Model file for the job. Use its own axes, mm. Round coordinates to 2 decimals unless told otherwise and drop trailing zeros. Loops run counter-clockwise (first coordinate to the right, second up) from the corner with the lowest first, then second, coordinate; pieces in that order, holes last. Notation, with made-up numbers: (44, 49) -> (80, 49) arc R13 ccw to (80, 69) -> close; hole circle Ø1 at (27, 66.25). An arc over 180 degrees is marked (long way). Use a Markdown table: item, result.
Autodesk Inventor part; units mm, degrees
ref_plane "YZ Plane" through (0, 0, 0) normal (1, 0, 0) x (0, 1, 0)
ref_plane "XZ Plane" through (0, 0, 0) normal (0, 1, 0) x (-1, 0, 0)
ref_plane "XY Plane" through (0, 0, 0) normal (0, 0, 1) x (1, 0, 0)
sketch "Sketch1" plane through (0, 0, 0) normal (0, 0, 1) x (1, 0, 0)
  line L0 (3.6662, -6.35) -> (-3.6662, -6.35)
  line L1 (-3.6662, -6.35) -> (-7.3323, 0)
  line L2 (-7.3323, 0) -> (-3.6662, 6.35)
  line L3 (-3.6662, 6.35) -> (3.6662, 6.35)
  line L4 (3.6662, 6.35) -> (7.3323, 0)
  line L5 (7.3323, 0) -> (3.6662, -6.35)
  point P0 (0, 0)
  point P1 (0, 0)
  dimension "d0" = 12.7
extrude "Extrusion1" add sketch "Sketch1" along normal blind 161.925
sketch "Sketch2" plane through (0, 0, 0) normal (0, 0, -1) x (-1, 0, 0)
  point P0 (0, 0)
  point P1 (0, 0)
hole "Hole1" at (0, 0, 0) direction (0, 0, 1) diameter 3.9624 depth 12.7 tip angle 118
properties part number "STOCK,HEX,SHAFT,HUB"
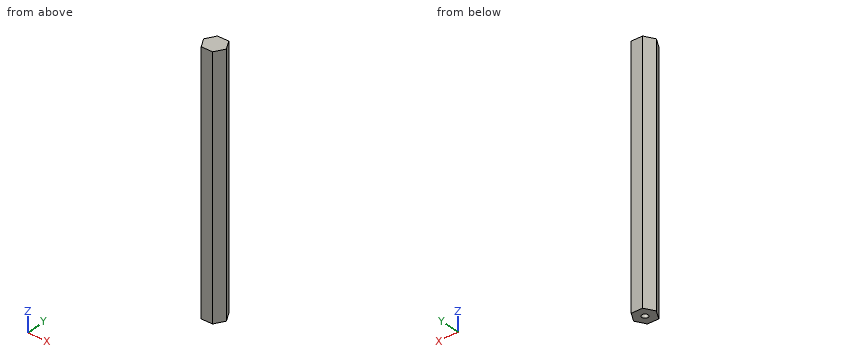
Q1. Flat gauge pins, fed straight in: pin 1 (5 mm diameter, centred on x = 0, y = 0, fed in from -Z); pin 2 (4 mm diameter, centred on y = 4, z = 60.5, fed in from +X). Where does each tip first touch, or does it go through?
Results list:
| item | result |
|---|---|
| pin 1 | stops at z = 0 |
| pin 2 | stops at x = 6.18 |
Q2. Drill centre lines: L1, parallel to Y at x = 0, z = 6; L2, parallel to X at y = 0, z = 9; L3, parallel to X at y = -5.5, z = 37.5. Where is each one in solid material? Low to high. Write a range as from..to.
Results list:
| item | result |
|---|---|
| L1 | y = -6.35..-1.98, 1.98..6.35 |
| L2 | x = -7.33..-1.98, 1.98..7.33 |
| L3 | x = -4.16..4.16 |
Q3. Band-saw the part on B-B, the plane x = 5.75. Give the cut face in (y, z) (3 decimals), plus the area to 3 significant figures.
Results list:
| item | result |
|---|---|
| outline | (-2.741, 0) -> (2.741, 0) -> (2.741, 161.925) -> (-2.741, 161.925) -> close |
| area | 888 mm² |
Q4. Band-saw the part on A-A, the plane z = 114. Give the cut face in (x, y).
Results list:
| item | result |
|---|---|
| outline | (-7.33, 0) -> (-3.67, -6.35) -> (3.67, -6.35) -> (7.33, 0) -> (3.67, 6.35) -> (-3.67, 6.35) -> close |
